Verification items for the finished model (mm, model axes). A direction names the side the tool comes from. Coordinates: 2 decimals unless noted, no trailing zeros. Order: outer loops, then holes, each group sorted by start corner. A loop starts at its lowest first (then second) coordinate and runs counter-clockwise, first axis right, second up. Notation, with made-up numbers: (-2.5, 20) -> (48.5, 20) arc R37 ccw to (48.5, 57) -> close; hole circle Ø8 at (7, 54.5). An arc over 180 degrees is marked (long way). Write item = value, one per line. Start each with the question number.
1. Cross-section at B-B on z = 2.65. Record the cut outline in (x, y) (3 decimals).
2. Cross-section at D-D on y = -43.5. Record the cut outline in (x, z) (3 decimals), plus the area to 3 significant figures.
3. Release check for a two-part mould opening along Y. For faces 3 (the cylindrical face through (11.6, -49.64, 2.03)), 4 (the flat face through (0, 50.5, 2)), 5 (the cylindrical face through (-0.704, -14.853, 1.972)) record: +Y half, -Y half, draft (parallel to the pull), parting line (faces both ways), or undercut.
4. Set-up check for faces 1 (the cylindrical face through (-0.1, 12.5, 2)), 2 (the cylindrical face through (-11.64, 49.6, 2.03)): record each of +Z, -Z, +X, -X, +Y, -Y from which the full face is reachable in a straight line by a thin tool's end or side.
5. Cross-section at A-A on y = -23.5. Record the cut outline in (x, z).
6. Cross-section at C-C on x = -0.25. Give the number of separate pieces and of enclosed holes in the cut face, plus the area to 3 significant figures.
7. Thickness scan on line 1 along X through (y, z) = (-43.5, 2.7) (3 decimals); line 2 along X through (y, z) = (3.5, 0.7). Record the ranges inside material, lowest first. Write a range as from..to.
from build123d import *

# Parameters (mm, degrees)
SKETCH_1_W               = 25
SKETCH_1_H               = 101
EXTRUDE_1_DEPTH          = 4
SKETCH_3_R               = 1.525
CUT_EXTRUDE_1_DEPTH      = 1
CUT_EXTRUDE_1_DEPTH_BACK = 5
FILLET_1_R               = 3
CUT_EXTRUDE_2_DEPTH      = 1
CUT_EXTRUDE_2_DEPTH_BACK = 5


with BuildPart() as part:
    # 草图1 → 凸台-拉伸1 (new body)
    with BuildSketch(Plane.XY):
        Rectangle(SKETCH_1_W, SKETCH_1_H)
    extrude(amount=EXTRUDE_1_DEPTH)

    # 草图3 → 切除-拉伸1 (cut, two sides)
    with BuildSketch(Plane(origin=(0, 0, 0), x_dir=(-1, 0, 0), z_dir=(0, 0, -1))) as cut_extrude_1_sk:
        with Locations((0, -43.500000001)):
            Circle(SKETCH_3_R)
        with Locations((0, -13.500000001)):
            Circle(SKETCH_3_R)
        with Locations((0, 16.499999999)):
            Circle(SKETCH_3_R)
        with Locations((0, 46.499999999)):
            Circle(SKETCH_3_R)
    extrude(amount=CUT_EXTRUDE_1_DEPTH, mode=Mode.SUBTRACT)
    extrude(cut_extrude_1_sk.sketch, amount=-CUT_EXTRUDE_1_DEPTH_BACK, mode=Mode.SUBTRACT)

    # 圆角1
    fillet_1_edges = [part.edges().sort_by_distance(p)[0] for p in [
        (12.5, -50.5, 2),
        (-12.5, -50.5, 2),
        (-12.5, 50.5, 2),
        (12.5, 50.5, 2),
    ]]
    fillet(fillet_1_edges, radius=FILLET_1_R)

    # 草图4 → 切除-拉伸2 (cut, two sides)
    with BuildSketch(Plane.XY.offset(4)) as cut_extrude_2_sk:
        with BuildLine():
            Line((-5, -34.500000001), (-5, -22.500000001))
            ThreePointArc((-5, -22.500000001), (0, -17.500000001), (5, -22.500000001))
            Line((5, -22.500000001), (5, -34.500000001))
            ThreePointArc((5, -34.500000001), (0, -39.500000001), (-5, -34.500000001))
        make_face()
        with BuildLine():
            Line((-5, -4.500000001), (-5, 7.499999999))
            ThreePointArc((-5, 7.499999999), (0, 12.499999999), (5, 7.499999999))
            Line((5, 7.499999999), (5, -4.500000001))
            ThreePointArc((5, -4.500000001), (0, -9.500000001), (-5, -4.500000001))
        make_face()
        with BuildLine():
            Line((-5, 25.499999999), (-5, 37.499999999))
            ThreePointArc((-5, 37.499999999), (0, 42.499999999), (5, 37.499999999))
            Line((5, 37.499999999), (5, 25.499999999))
            ThreePointArc((5, 25.499999999), (0, 20.499999999), (-5, 25.499999999))
        make_face()
    extrude(amount=CUT_EXTRUDE_2_DEPTH, mode=Mode.SUBTRACT)
    extrude(cut_extrude_2_sk.sketch, amount=-CUT_EXTRUDE_2_DEPTH_BACK, mode=Mode.SUBTRACT)


solid = part.part
Worked out:
q1.outline = (-12.5, -47.5) arc R3 ccw to (-9.5, -50.5) -> (9.5, -50.5) arc R3 ccw to (12.5, -47.5) -> (12.5, 47.5) arc R3 ccw to (9.5, 50.5) -> (-9.5, 50.5) arc R3 ccw to (-12.5, 47.5) -> close; hole (-5, -34.5) arc R5 ccw to (5, -34.5) -> (5, -22.5) arc R5 ccw to (-5, -22.5) -> close; hole (-5, -4.5) arc R5 ccw to (5, -4.5) -> (5, 7.5) arc R5 ccw to (-5, 7.5) -> close; hole (-5, 25.5) arc R5 ccw to (5, 25.5) -> (5, 37.5) arc R5 ccw to (-5, 37.5) -> close; hole circle Ø3.05 at (0, -43.5); hole circle Ø3.05 at (0, -13.5); hole circle Ø3.05 at (0, 16.5); hole circle Ø3.05 at (0, 46.5)
q2.outline = (-12.5, 0) -> (-1.525, 0) -> (-1.525, 4) -> (-12.5, 4) -> close; (1.525, 0) -> (12.5, 0) -> (12.5, 4) -> (1.525, 4) -> close
q2.area = 87.8 mm²
q3.face_3 = -Y half
q3.face_4 = +Y half
q3.face_5 = undercut
q4.face_1 = +Z, -Z
q4.face_2 = +Z, -Z, -X, +Y
q5.outline = (-12.5, 0) -> (-5, 0) -> (-5, 4) -> (-12.5, 4) -> close; (5, 0) -> (12.5, 0) -> (12.5, 4) -> (5, 4) -> close
q6.separate_pieces = 8
q6.enclosed_holes = 0
q6.area = 92.0 mm²
q7.line_1 = -12.5..-1.525, 1.525..12.5
q7.line_2 = -12.5..-5, 5..12.5
